For this review, take the finished solid that the model builds, in its own axes (mm). Give positions to 0.01 mm unless a question says otherwise; leave off trailing zeros. Write each loop counter-clockwise with the first axis right and the second up, starting at its lowest first coordinate (ties: lowest second). Pieces come first, ordered by that corner, then holes. Notation, with made-up numbers: M 46,44 L 67,44 A17 cw 67,55 Z; hole C -18,35.5 d9. An arc over 180 degrees is marked long. Use one line per item in the form item = value. Start each with the question number.
Q1. Clearance check with a flat-ended pin moving along its axis: pin 1 Ø5 at (x, z) = (395, 5) entering from -Y. State where the tip first meets the part, or that it passes through.
Q2. Consider section A-A on z = 0. Write out the cut boundary in (x, y), and give its area (3 significant figures).
Q3. Consider section B-B on x = -279. Write out the cut boundary in (y, z), and give its area (3 significant figures).
Q4. For probe 1 along X at (y, z) = (1.55, 0.5); probe 2 along Z at (x, y) = (193.5, -0.8); probe 3 along X at (y, z) = (0.8, 1), list the stretches that pass through material, from the lowest coordinate up. Write a range as [from, to].
Solid Edge part; units mm, degrees
sketch "Sketch1" plane through (0, 0, 0) normal (0, -1, 0) x (1, 0, 0)
  arc A0 (490, -8) -> (490, 8) centre (490, 0) ccw
  line L0 (490, 8) -> (-490, 8)
  arc A1 (-490, 8) -> (-490, -8) centre (-490, 0) ccw
  line L1 (-490, -8) -> (490, -8)
  line L2 (-490, -6) -> (490, -6)
  arc A2 (-490, 6) -> (-490, -6) centre (-490, 0) ccw
  line L3 (490, 6) -> (-490, 6)
  arc A3 (490, -6) -> (490, 6) centre (490, 0) ccw
  dimension "D1" = 490
extrude "Protrusion1" add sketch "Sketch1" along normal mid plane 5
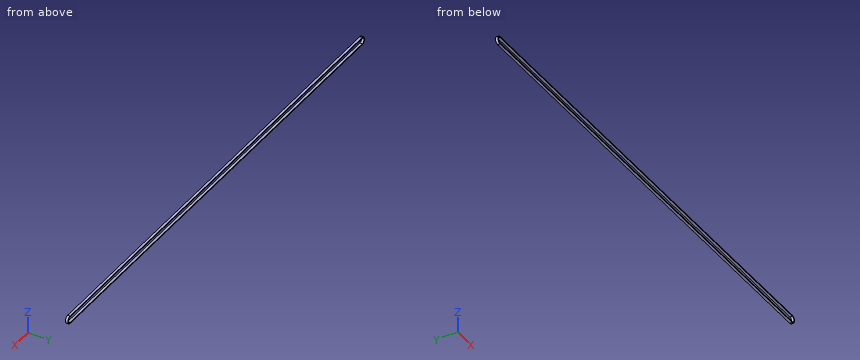
Working result:
q1.pin_1 = -2.5
q2.outline = M -498,-2.5 L -496,-2.5 L -496,2.5 L -498,2.5 Z; M 496,-2.5 L 498,-2.5 L 498,2.5 L 496,2.5 Z
q2.area = 20.0 mm²
q3.outline = M -2.5,-8 L 2.5,-8 L 2.5,-6 L -2.5,-6 Z; M -2.5,6 L 2.5,6 L 2.5,8 L -2.5,8 Z
q3.area = 20.0 mm²
q4.probe_1 = [-497.98, -495.98], [495.98, 497.98]
q4.probe_2 = [-8, -6], [6, 8]
q4.probe_3 = [-497.94, -495.92], [495.92, 497.94]
